The model under review builds one solid part; all positions refer to its coordinate system, in mm. Face numbers are marked on the shaded views. Round coordinates to 2 decimals unless told otherwise and drop trailing zeros. Write each loop counter-clockwise with the first axis right and the second up, starting at its lowest first coordinate (ties: lowest second). Pieces come first, ordered by that corner, then holes. Notation, with made-up numbers: (-39.5, -6.75) - (-8.5, -6.75) arc R11 ccw to (-8.5, -2.75) - close; hole circle Ø9 at (-25, 31). An arc over 180 degrees is marked (long way). Write each question's results on one line, items separated by ' | '.
```python
from build123d import *

# Parameters (mm, degrees)
BOSS_EXTRUDE1_DEPTH = 12.5
CUT_EXTRUDE1_START  = 12.5
SKETCH4_R           = 5
CUT_EXTRUDE1_DEPTH  = 9.3
BOSS_EXTRUDE2_START = 12.5
SKETCH6_R           = 35
BOSS_EXTRUDE2_DEPTH = 7.5
CUT_EXTRUDE5_START  = 20
SKETCH9_R           = 2.55
CUT_EXTRUDE5_DEPTH  = 12
SKETCH5_R           = 2.05
CUT_EXTRUDE6_DEPTH  = 10


with BuildPart() as part:
    # Sketch2 → Boss-Extrude1 (new body)
    with BuildSketch(Plane(origin=(0, 0, 0), x_dir=(0, 1, 0), z_dir=(0, 0, 1))):
        with BuildLine():
            ThreePointArc((3.402279768, 20.103447736), (0, 22), (-3.402279768, 20.103447736))
            ThreePointArc((-3.402279768, 20.103447736), (-7.622462843, 15.658643671), (-13.268220181, 13.272925238))
            ThreePointArc((-13.268220181, 13.272925238), (-14.482955544, 13.085514107), (-15.708956559, 12.998184578))
            ThreePointArc((-15.708956559, 12.998184578), (-19.052558883, 11), (-19.111236327, 7.105263158))
            ThreePointArc((-19.111236327, 7.105263158), (-17.775931243, 3.663582804), (-17.321657799, 0))
            ThreePointArc((-17.321657799, 0), (-17.775931243, -3.663582804), (-19.111236327, -7.105263158))
            ThreePointArc((-19.111236327, -7.105263158), (-19.052558883, -11), (-15.708956559, -12.998184578))
            ThreePointArc((-15.708956559, -12.998184578), (-14.482955544, -13.085514107), (-13.268220181, -13.272925238))
            ThreePointArc((-13.268220181, -13.272925238), (-7.622462843, -15.658643671), (-3.402279768, -20.103447736))
            ThreePointArc((-3.402279768, -20.103447736), (0, -22), (3.402279768, -20.103447736))
            ThreePointArc((3.402279768, -20.103447736), (7.622462843, -15.658643671), (13.268220181, -13.272925238))
            ThreePointArc((13.268220181, -13.272925238), (14.482955544, -13.085514107), (15.708956559, -12.998184578))
            ThreePointArc((15.708956559, -12.998184578), (19.052558883, -11), (19.111236327, -7.105263158))
            ThreePointArc((19.111236327, -7.105263158), (17.775931243, -3.663582804), (17.321657799, 0))
            ThreePointArc((17.321657799, 0), (17.775931243, 3.663582804), (19.111236327, 7.105263158))
            ThreePointArc((19.111236327, 7.105263158), (19.052558883, 11), (15.708956559, 12.998184578))
            ThreePointArc((15.708956559, 12.998184578), (9.749551787, 14.430568297), (4.860580348, 18.127078359))
            ThreePointArc((4.860580348, 18.127078359), (4.090909866, 19.085364477), (3.402279768, 20.103447736))
        make_face()
    extrude(amount=BOSS_EXTRUDE1_DEPTH)

    # Sketch4 → Cut-Extrude1 (cut)
    with BuildSketch(Plane(origin=(0, 0, 0), x_dir=(0, 1, 0), z_dir=(0, 0, 1)).offset(CUT_EXTRUDE1_START)):
        with Locations((-15.588457268, 9)):
            Circle(SKETCH4_R)
        with Locations((0, 18)):
            Circle(SKETCH4_R)
        with Locations((15.588457268, 9)):
            Circle(SKETCH4_R)
        with Locations((15.588457268, -9)):
            Circle(SKETCH4_R)
        with Locations((0, -18)):
            Circle(SKETCH4_R)
        with Locations((-15.588457268, -9)):
            Circle(SKETCH4_R)
    extrude(amount=-CUT_EXTRUDE1_DEPTH, mode=Mode.SUBTRACT)

    # Sketch6 → Boss-Extrude2 (add)
    with BuildSketch(Plane(origin=(0, 0, 0), x_dir=(0, 1, 0), z_dir=(0, 0, 1)).offset(BOSS_EXTRUDE2_START)):
        with Locations(Location((0, 0, 0), (0, 0, 270))):
            Circle(SKETCH6_R)
    extrude(amount=BOSS_EXTRUDE2_DEPTH)

    # Sketch9 → Cut-Extrude5 (cut)
    with BuildSketch(Plane(origin=(0, 0, 0), x_dir=(0, 1, 0), z_dir=(0, 0, 1)).offset(CUT_EXTRUDE5_START)):
        with Locations(Location((12.5, 21.650635095, 0), (0, 0, 270))):
            Circle(SKETCH9_R)
        with Locations(Location((25, 0, 0), (0, 0, 270))):
            Circle(SKETCH9_R)
        with Locations(Location((12.5, -21.650635095, 0), (0, 0, 270))):
            Circle(SKETCH9_R)
        with Locations(Location((-12.5, -21.650635095, 0), (0, 0, 270))):
            Circle(SKETCH9_R)
        with Locations(Location((-25, 0, 0), (0, 0, 270))):
            Circle(SKETCH9_R)
        with Locations(Location((-12.5, 21.650635095, 0), (0, 0, 270))):
            Circle(SKETCH9_R)
    extrude(amount=-CUT_EXTRUDE5_DEPTH, mode=Mode.SUBTRACT)

    # Sketch5 → Cut-Extrude6 (cut)
    with BuildSketch(Plane(origin=(0, 0, 0), x_dir=(0, 1, 0), z_dir=(0, 0, 1))):
        with Locations(Location((-15.588457268, 9, 0), (0, 0, 270))):
            Circle(SKETCH5_R)
        with Locations(Location((0, 18, 0), (0, 0, 270))):
            Circle(SKETCH5_R)
        with Locations(Location((15.588457268, 9, 0), (0, 0, 270))):
            Circle(SKETCH5_R)
        with Locations(Location((15.588457268, -9, 0), (0, 0, 270))):
            Circle(SKETCH5_R)
        with Locations(Location((0, -18, 0), (0, 0, 270))):
            Circle(SKETCH5_R)
        with Locations(Location((-15.588457268, -9, 0), (0, 0, 270))):
            Circle(SKETCH5_R)
    extrude(amount=CUT_EXTRUDE6_DEPTH, mode=Mode.SUBTRACT)


solid = part.part
```
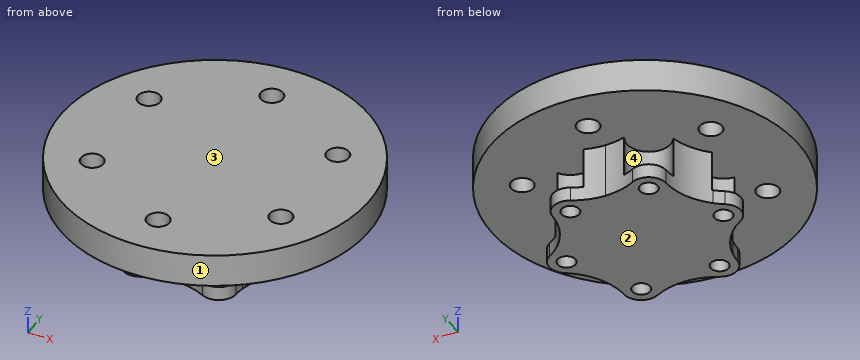
Q1. We need section B-B (x = -9). State the section outline as (y, z) points, plus the area to 3 significant figures.
Evaluation:
outline: (-33.82, 12.5) - (-10.59, 12.5) - (-10.59, 3.2) - (-13.54, 3.2) - (-13.54, 0) - (13.54, 0) - (13.54, 3.2) - (10.59, 3.2) - (10.59, 12.5) - (33.82, 12.5) - (33.82, 20) - (-33.82, 20) - close; (-19.59, 0) - (-17.64, 0) - (-17.64, 3.2) - (-19.59, 3.2) - close; (17.64, 0) - (19.59, 0) - (19.59, 3.2) - (17.64, 3.2) - close | area: 803 mm^2
Q2. Insertion check: P1, Ø2, axis at x = -21.5, z = 3, coming from the -Y side; P2, Ø6.5, axis at x = 21.65, y = -12.5, coming from the +Z side; P3, Ø3, axis at x = 27.5, y = -8.5, coming from the -Z side; P4, Ø10, axis at y = -14, z = 15.5, coming from the -X side. Each pin has a flat end and moves straight along its axis. Give the tip position at first contact, or say it passes through.
Evaluation:
P1: stops at y = -3.12 | P2: stops at z = 20 | P3: stops at z = 12.5 | P4: stops at x = -33.82
Q3. The part is to be moulded in two halves that separate along Z. For the marked faces 1, 2, 3 and 4, say which applies: released by +Z, released by -Z, zero draft, split by the parting line, or undercut.
Evaluation:
face 1: zero draft | face 2: released by -Z | face 3: released by +Z | face 4: undercut
Q4. We need section A-A (y = 0). State the section outline as (x, z) points, plus the area to 3 significant figures.
Evaluation:
outline: (-35, 12.5) - (-13, 12.5) - (-13, 3.2) - (-15.95, 3.2) - (-15.95, 0) - (15.95, 0) - (15.95, 3.2) - (13, 3.2) - (13, 12.5) - (35, 12.5) - (35, 20) - (-35, 20) - close; (-22, 0) - (-20.05, 0) - (-20.05, 3.2) - (-22, 3.2) - close; (20.05, 0) - (22, 0) - (22, 3.2) - (20.05, 3.2) - close | area: 881 mm^2
Q5. We need section D-D (y = -25). State the section outline as (x, z) points.
Evaluation:
outline: (-24.49, 12.5) - (-2.55, 12.5) - (-2.55, 20) - (-24.49, 20) - close; (2.55, 12.5) - (24.49, 12.5) - (24.49, 20) - (2.55, 20) - close
Q6. We need section C-C (z = 2.25). State the section outline as (x, y) points, plus the area to 3 significant figures.
Evaluation:
outline: (-20.1, -3.4) arc R15 cw to (-13, -15.71) arc R4 ccw to (-7.11, -19.11) arc R15 cw to (7.11, -19.11) arc R4 ccw to (13, -15.71) arc R15 cw to (20.1, -3.4) arc R4 ccw to (20.1, 3.4) arc R15 cw to (13, 15.71) arc R4 ccw to (7.11, 19.11) arc R15 cw to (-7.11, 19.11) arc R4 ccw to (-13, 15.71) arc R15 cw to (-20.1, 3.4) arc R4 ccw to start; hole circle Ø4.1 at (-18, 0); hole circle Ø4.1 at (-9, -15.59); hole circle Ø4.1 at (-9, 15.59); hole circle Ø4.1 at (9, -15.59); hole circle Ø4.1 at (9, 15.59); hole circle Ø4.1 at (18, 0) | area: 1,100 mm^2
Q7. For probe 1 along Y at (x, z) = (-9, 1.5); probe 2 along X at (y, z) = (0, 1.95); probe 3 along X at (y, z) = (-11, 16), list the stretches that pass through material, from the lowest coordinate up.
Evaluation:
probe 1: y = -19.59 to -17.64, -13.54 to 13.54, 17.64 to 19.59 | probe 2: x = -22 to -20.05, -15.95 to 15.95, 20.05 to 22 | probe 3: x = -33.23 to -23.71, -19.59 to 19.59, 23.71 to 33.23
